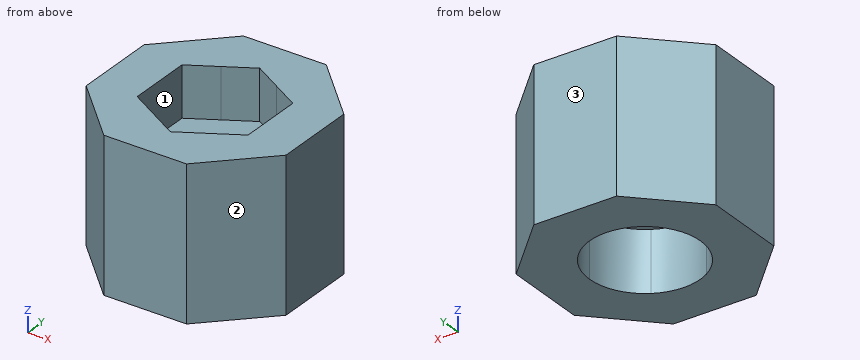
```python
from build123d import *

# Parameters (mm, degrees)
F1_DEPTH = 7.5
F2_DEPTH = 5
F0_R     = 1.5
F3_DEPTH = 5
F4_DEPTH = 3


with BuildPart() as f1:
    # F0 (on Top) → F1 (new body)
    with BuildSketch(Plane.XY):
        Polygon((2.0535090273, 4.9576093443), (-2.0535090273, 4.9576093443), (-4.9576093443, 2.0535090273), (-4.9576093443, -2.0535090273), (-2.0535090273, -4.9576093443), (2.0535090273, -4.9576093443), (4.9576093443, -2.0535090273), (4.9576093443, 2.0535090273), align=None)
        Polygon((2.75, 1.5877132403), (2.75, 0), (2.75, -1.5877132403), (1.3750001046, -2.3815698), (0, -3.1754264805), (-1.3750000168, -2.3815698507), (-2.75, -1.5877132403), (-2.75, 0), (-2.75, 1.5877132403), (-1.3749999907, 2.3815698658), (0, 3.1754264805), (1.3750000803, 2.381569814), align=None, mode=Mode.SUBTRACT)
    extrude(amount=F1_DEPTH)

    # F0 (on Top) → F2 (join)
    with BuildSketch(Plane.XY):
        with BuildLine():
            ThreePointArc((-2.75, 0), (-2.3815698577, 1.3750000046), (-1.3749999907, 2.3815698658))
            Line((-1.3749999907, 2.3815698658), (-2.75, 1.5877132403))
            Line((-2.75, 1.5877132403), (-2.75, 0))
        make_face()
        with BuildLine():
            ThreePointArc((-1.3749999907, 2.3815698658), (5.17e-08, 2.75), (1.3750000803, 2.381569814))
            Line((1.3750000803, 2.381569814), (0, 3.1754264805))
            Line((0, 3.1754264805), (-1.3749999907, 2.3815698658))
        make_face()
        with BuildLine():
            ThreePointArc((1.3750000803, 2.381569814), (2.3815698836, 1.3749999598), (2.75, 0))
            Line((2.75, 0), (2.75, 1.5877132403))
            Line((2.75, 1.5877132403), (1.3750000803, 2.381569814))
        make_face()
        with BuildLine():
            Line((2.75, -1.5877132403), (2.75, 0))
            ThreePointArc((2.75, 0), (2.3815698906, -1.3749999477), (1.3750001046, -2.3815698))
            Line((1.3750001046, -2.3815698), (2.75, -1.5877132403))
        make_face()
        with BuildLine():
            Line((0, -3.1754264805), (1.3750001046, -2.3815698))
            ThreePointArc((1.3750001046, -2.3815698), (5.07e-08, -2.75), (-1.3750000168, -2.3815698507))
            Line((-1.3750000168, -2.3815698507), (0, -3.1754264805))
        make_face()
        with BuildLine():
            Line((-2.75, -1.5877132403), (-1.3750000168, -2.3815698507))
            ThreePointArc((-1.3750000168, -2.3815698507), (-2.3815698653, -1.3749999916), (-2.75, 0))
            Line((-2.75, 0), (-2.75, -1.5877132403))
        make_face()
    extrude(amount=F2_DEPTH)

    # F0 (on Top) → F3 (join)
    with BuildSketch(Plane.XY):
        with BuildLine():
            ThreePointArc((1.3750001046, -2.3815698), (2.3815698906, -1.3749999477), (2.75, 0))
            ThreePointArc((2.75, 0), (2.3815698836, 1.3749999598), (1.3750000803, 2.381569814))
            ThreePointArc((1.3750000803, 2.381569814), (5.17e-08, 2.75), (-1.3749999907, 2.3815698658))
            ThreePointArc((-1.3749999907, 2.3815698658), (-2.3815698577, 1.3750000046), (-2.75, 0))
            ThreePointArc((-2.75, 0), (-2.3815698653, -1.3749999916), (-1.3750000168, -2.3815698507))
            ThreePointArc((-1.3750000168, -2.3815698507), (5.07e-08, -2.75), (1.3750001046, -2.3815698))
        make_face()
        Circle(F0_R, mode=Mode.SUBTRACT)
    extrude(amount=F3_DEPTH)

    # F0 (on Top) → F4 (cut)
    with BuildSketch(Plane.XY):
        with BuildLine():
            ThreePointArc((1.3750001046, -2.3815698), (2.3815698906, -1.3749999477), (2.75, 0))
            ThreePointArc((2.75, 0), (2.3815698836, 1.3749999598), (1.3750000803, 2.381569814))
            ThreePointArc((1.3750000803, 2.381569814), (5.17e-08, 2.75), (-1.3749999907, 2.3815698658))
            ThreePointArc((-1.3749999907, 2.3815698658), (-2.3815698577, 1.3750000046), (-2.75, 0))
            ThreePointArc((-2.75, 0), (-2.3815698653, -1.3749999916), (-1.3750000168, -2.3815698507))
            ThreePointArc((-1.3750000168, -2.3815698507), (5.07e-08, -2.75), (1.3750001046, -2.3815698))
        make_face()
        Circle(F0_R, mode=Mode.SUBTRACT)
    extrude(amount=F4_DEPTH, mode=Mode.SUBTRACT)


solid = f1.part
```
Could you check a few things on this model? Use its own coordinates, in mm. Face numbers are marked on the shaded views. Round coordinates to 2 decimals unless told otherwise and drop trailing zeros. Loops run counter-clockwise (first coordinate to the right, second up) from the corner with the lowest first, then second, coordinate; pieces in that order, holes last.
Q1. I want a section at B-B (y = 0.5). Write out the boundary of the cut face in (x, z), and give its area (3 significant figures).
Q2. I want a section at D-D (z = 4.75). Write out the boundary of the cut face in (x, y), and give its area (3 significant figures).
Q3. I want a section at C-C (x = 2.5). Write out the boundary of the cut face in (y, z), and give its area (3 significant figures).
Q4. Please list where these lines run through material, in increasing order: L1, parallel to Y at x = 0, z = 4.1; L2, parallel to X at y = 1.5, z = 5.25; L3, parallel to Z at x = -0.75, y = -2.
Q5. Thinking about a two-plate mould opening in X: for the marked faces 1, 2 and 3, which applies, pulls with the +X half, pulls with the -X half, needs draft (parallel to the pull), parting line crosses it, or undercut?
Q6. For P1, Ø5, axis at x = 0, y = 0, coming from the +Z side; P2, Ø3, axis at x = 2.5, z = 3, coming from the -Y side; P3, Ø1.6, axis at x = 0.5, y = -1, coming from the -Z side, each with a flat end and sliding along its axis, tell me the tip position at first contact or that it passes through.
Answer below:
1. outline: (-4.96, 0) - (-2.7, 0) - (-2.7, 3) - (-1.41, 3) - (-1.41, 5) - (-2.75, 5) - (-2.75, 7.5) - (-4.96, 7.5) - close; (1.41, 3) - (2.7, 3) - (2.7, 0) - (4.96, 0) - (4.96, 7.5) - (2.75, 7.5) - (2.75, 5) - (1.41, 5) - close
1. area: 38.7 mm2
2. outline: (-4.96, -2.05) - (-2.05, -4.96) - (2.05, -4.96) - (4.96, -2.05) - (4.96, 2.05) - (2.05, 4.96) - (-2.05, 4.96) - (-4.96, 2.05) - close; hole circle Ø3 at (0, 0)
2. area: 74.4 mm2
3. outline: (-4.51, 0) - (-1.15, 0) - (-1.15, 3) - (1.15, 3) - (1.15, 0) - (4.51, 0) - (4.51, 7.5) - (1.73, 7.5) - (1.73, 5) - (-1.73, 5) - (-1.73, 7.5) - (-4.51, 7.5) - close
3. area: 52.1 mm2
4. L1: y = -4.96 to -1.5, 1.5 to 4.96
4. L2: x = -4.96 to -2.75, 2.75 to 4.96
4. L3: z = 3 to 5
5. face 1: undercut
5. face 2: pulls with the +X half
5. face 3: needs draft
6. P1: stops at z = 5
6. P2: stops at y = -4.96
6. P3: stops at z = 3
